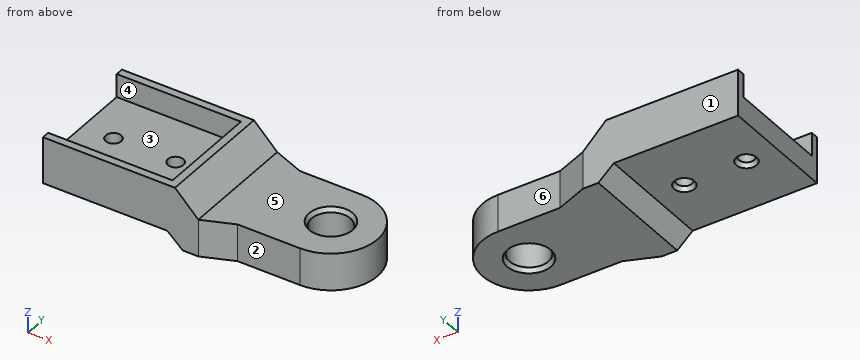
Solid Edge part; units mm, degrees
sketch "Sketch1" plane through (0, 0, 0) normal (0, -1, 0) x (1, 0, 0)
  line L0 (-40, 15) -> (-40, 0)
  line L1 (-40, 0) -> (0, 0)
  line L2 (0, 0) -> (5, -4.5)
  line L3 (5, -4.5) -> (60, -4.5)
  line L4 (60, -4.5) -> (60, 7.5)
  line L5 (60, 7.5) -> (10, 7.5)
  line L6 (10, 7.5) -> (10, 15)
  line L7 (10, 15) -> (-40, 15)
  dimension "D1" = 40
  dimension "D2" = 10
  dimension "D3" = 10
  dimension "D4" = 60
  dimension "D5" = 60
extrude "Protrusion1" add sketch "Sketch1" along normal mid plane 38
sketch "Sketch2" plane through (-15, 0, 15) normal (0, 0, 1) x (1, 0, 0)
  line L0 (-25, 16.5) -> (15, 16.5)
  line L1 (15, 16.5) -> (15, -16.5)
  line L2 (15, -16.5) -> (-25, -16.5)
  line L3 (-25, -16.5) -> (-25, 16.5)
  dimension "D1" = 25
extrude "ExtrudedCutout_1" cut sketch "Sketch2" against normal blind 7.5
hole "Hole_1" at (-10, 0, 7.5) direction (0, 0, -1) diameter 5 end up to next
hole "Hole1" at (-30, 0, 7.5) direction (0, 0, -1) diameter 5 end up to next
hole "Hole_3" at (40, 0, 7.5) direction (0, 0, -1) diameter 12.5 end up to next
sketch "Sketch3" plane through (35, 0, 7.5) normal (0, 0, 1) x (-1, 0, 0)
  line L0 (15, -15) -> (25, -19)
  line L1 (-5, -15) -> (15, -15)
  arc A0 (-5, 15) -> (-5, -15) centre (-5, 0) ccw
  line L2 (-5, 15) -> (15, 15)
  line L3 (15, 15) -> (25, 19)
  dimension "D1" = 20
  dimension "D2" = 15
extrude "Cutout1" cut sketch "Sketch3" against normal through all material side at (15.0186, 17.0464, 7.5)
chamfer "Chamfer_1" distance 7.5 angle 45 1 edges at (10, 0, 15)
chamfer "Chamfer_2" distance 0.8 angle 60 4 edges at (33.75, 0, -4.5) (46.25, 0, 7.5) (-12.5, 0, 0) (-32.5, 0, 0) measured on face at (47.95, -12.2867, 7.5) measured on face at (12.8333, -12.2867, -4.5) measured on face at (-33.7333, -12.2867, 0)
properties material "Polyethylene, low density"
The model under review builds one solid part; all positions refer to its coordinate system, in mm. Face numbers are marked on the shaded views. A direction names the side the tool comes from. Coordinates: 2 decimals unless noted, no trailing zeros. Order: outer loops, then holes, each group sorted by start corner. A loop starts at its lowest first (then second) coordinate and runs counter-clockwise, first axis right, second up. Notation, with made-up numbers: (-34.75, 5.25) -> (4.25, 5.25) arc R27 ccw to (4.25, 39.25) -> close; hole circle Ø7 at (69, 79). An arc over 180 degrees is marked (long way). Answer in a Markdown table with one row per item. Add a question column.
Item 1: We need section B-B on x = -10. Write out the cut boundary in (y, z).
Item 2: Clearance check with flat-ended pins moving along their axes: pin 1 (1 mm diameter, centred on x = 39.5, z = -2.5, fed in from +Y); pin 2 (19 mm diameter, centred on x = -15.5, y = 6.5, fed in from -Z); pin 3 (8 mm diameter, centred on x = 15.5, z = 6.5, fed in from +Y). State where each tip first meets the part, or that it passes through.
Item 3: Mouldability with a two-part tool opening along Y and no side actions: class the marked faces 1, 2 and 3 as +Y half, -Y half, draft (parallel to the pull), parting line (faces both ways), or undercut.
Item 4: Machinability: for the marked faces 4, 5 and 6, which of the approach directions +Z, -Z, +X, -X, +Y, -Y give a long, thin tool a straight path to every point of the face, cutting with its end or side? Answer none if there is none.
Item 5: We need section A-A on y = 0. Give the number of separate pieces and of enclosed holes in the cut face, plus the area to 3 significant figures.
Item 6: We need section D-D on z = -2. Write out the cut boundary in (x, y).
Item 7: We need section C-C on z = 2.5. Write out the cut boundary in (x, y), plus the area to 3 significant figures.
Item 8: To check wall thickness, follow probe 1 along X at (y, z) = (0, 4); probe 2 along Y at (x, z) = (-10, 4.25); probe 3 along X at (y, z) = (1, 6.25). State the ranges of each line that lie inside material, in increasing order.
Final values:
| question | item | result |
|---|---|---|
| 1 | outline | (-19, 0) -> (-3.3, 0) -> (-2.5, 1.39) -> (-2.5, 7.5) -> (-16.5, 7.5) -> (-16.5, 15) -> (-19, 15) -> close; (2.5, 1.39) -> (3.3, 0) -> (19, 0) -> (19, 15) -> (16.5, 15) -> (16.5, 7.5) -> (2.5, 7.5) -> close |
| 2 | pin 1 | stops at y = 15 |
| 2 | pin 2 | stops at z = 0 |
| 2 | pin 3 | stops at y = 18.4 |
| 3 | face 1 | +Y half |
| 3 | face 2 | -Y half |
| 3 | face 3 | undercut |
| 4 | face 4 | +Z, -X |
| 4 | face 5 | +Z, +X, +Y, -Y |
| 4 | face 6 | +Z, -Z, +X, +Y |
| 5 | separate pieces | 4 |
| 5 | enclosed holes | 0 |
| 5 | area | 766 mm2 |
| 6 | outline | (2.22, -19) -> (10, -19) -> (20, -15) -> (40, -15) arc R15 ccw to (40, 15) -> (20, 15) -> (10, 19) -> (2.22, 19) -> close; hole circle Ø12.5 at (40, 0) |
| 7 | outline | (-40, -19) -> (10, -19) -> (20, -15) -> (40, -15) arc R15 ccw to (40, 15) -> (20, 15) -> (10, 19) -> (-40, 19) -> close; hole circle Ø5 at (-30, 0); hole circle Ø5 at (-10, 0); hole circle Ø12.5 at (40, 0) |
| 7 | area | 3,030 mm2 |
| 8 | probe 1 | x = -40 to -32.5, -27.5 to -12.5, -7.5 to 33.75, 46.25 to 55 |
| 8 | probe 2 | y = -19 to -2.5, 2.5 to 19 |
| 8 | probe 3 | x = -40 to -32.29, -27.71 to -12.29, -7.71 to 33.75, 46.25 to 54.97 |
